Geometry check sheet. Reference: drawing and pictorial views, mm from the part's lowest x, y, z. A direction names the side the tool comes from. Round coordinates to 2 decimals unless told otherwise and drop trailing zeros. Order: outer loops, then holes, each group sorted by start corner. A loop starts at its lowest first (then second) coordinate and runs counter-clockwise, first axis right, second up.
(1) Sectioned sample at A-A (z = 12.7). Record the boundary of the cut face in (x, y) (1 decimal), plus the area to 3 significant figures.
(2) Go/stop test with flat-tipped pins: pin 1 (12.5 mm diameter, centred on y = 34, z = 6.5, fed in from +X) (1 decimal); pin 2 (2.5 mm diameter, centred on y = 49, z = 19, fed in from +X); pin 3 (3 mm diameter, centred on x = 52.96, z = 5.26, fed in from +Y) (1 decimal); pin 4 (9 mm diameter, centred on x = 52.959, z = 12.7, fed in from +Y). Record where each tip stops, or that it passes through.
(3) Material ranges on line 1 along Y through (x, z) = (8.5, 20.25) (1 decimal); line 2 along X through (y, z) = (1, 12.7) (1 decimal); line 3 along Y through (x, z) = (38.5, 22) (1 decimal), recorded low to high.
(4) Set-up check for the marked faces 1 and 2: record each of +Z, -Z, +X, -X, +Y, -Y from which the full face is reachable in a straight line by a thin tool's end or side.
(5) Sectioned sample at B-B (x = 50). Record the boundary of the cut face in (y, z) (1 decimal).
(6) Release check for a two-part mould opening along Y. For the marked faces 3, 4 and 5 record: +Y half, -Y half, draft (parallel to the pull), parting line (faces both ways), or undercut.
(7) Sectioned sample at C-C (y = 20). Record the boundary of the cut face in (x, z) (1 decimal).
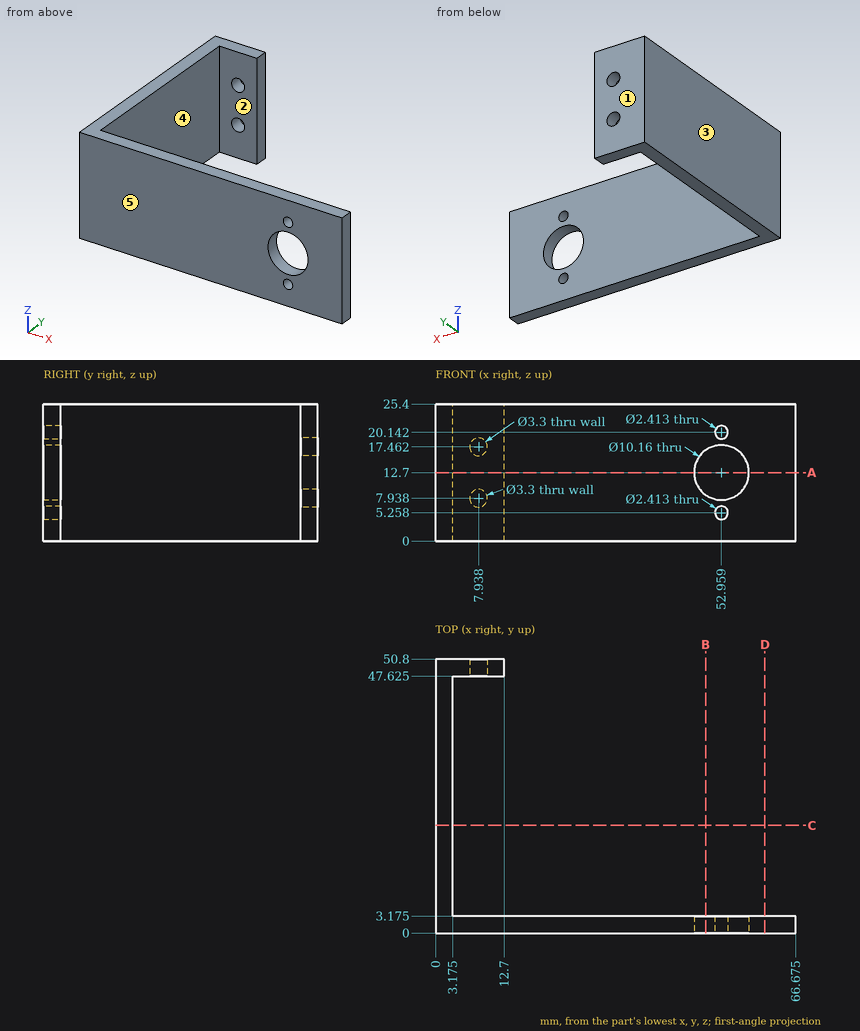
Answer below:
1. outline: (0, 0) - (47.9, 0) - (47.9, 3.2) - (3.2, 3.2) - (3.2, 47.6) - (12.7, 47.6) - (12.7, 50.8) - (0, 50.8) - close; (58, 0) - (66.7, 0) - (66.7, 3.2) - (58, 3.2) - close
1. area: 361 mm2
2. pin 1: stops at x = 3.2
2. pin 2: stops at x = 12.7
2. pin 3: stops at y = 3.2
2. pin 4: passes through
3. line 1: y = 0 to 3.2, 47.6 to 50.8
3. line 2: x = 0 to 47.9, 58 to 66.7
3. line 3: y = 0 to 3.2
4. face 1: +Z, -Z, +X, -X, +Y
4. face 2: +Z, -Z, +X
5. outline: (0, 0) - (3.2, 0) - (3.2, 8.6) - (0, 8.6) - close; (0, 16.8) - (3.2, 16.8) - (3.2, 25.4) - (0, 25.4) - close
6. face 3: draft
6. face 4: undercut
6. face 5: -Y half
7. outline: (0, 0) - (3.2, 0) - (3.2, 25.4) - (0, 25.4) - close
